```python
from build123d import *

# Parameters (mm, degrees)
SKETCH_1_R      = 1.75
SKETCH_1_R_2    = 1
EXTRUDE_1_DEPTH = 2.5
SKETCH_3_W      = 0.75
SKETCH_3_H      = 10
EXTRUDE_2_DEPTH = 0.75
SKETCH_4_W      = 10
SKETCH_4_H      = 0.75
EXTRUDE_3_DEPTH = 0.75


with BuildPart() as part:
    # 草图1 → 凸台-拉伸1 (new, symmetric)
    with BuildSketch(Plane.XY):
        Circle(SKETCH_1_R)
        Circle(SKETCH_1_R_2, mode=Mode.SUBTRACT)
    extrude(amount=EXTRUDE_1_DEPTH, both=True)

    # 草图3 → 凸台-拉伸2 (add)
    with BuildSketch(Plane.XY.offset(2.5)):
        with Locations((-1.375, -5)):
            Rectangle(SKETCH_3_W, SKETCH_3_H)
    extrude(amount=-EXTRUDE_2_DEPTH)

    # 草图4 → 凸台-拉伸3 (add)
    with BuildSketch(Plane(origin=(0, 0, -2.5), x_dir=(-1, 0, 0), z_dir=(0, 0, -1))):
        with Locations((-5, 1.375)):
            Rectangle(SKETCH_4_W, SKETCH_4_H)
    extrude(amount=-EXTRUDE_3_DEPTH)


solid = part.part
```
Work out the finished part from the listing and answer in its coordinate system (mm). Give positions to 0.01 mm unless a question says otherwise; leave off trailing zeros. Order: outer loops, then holes, each group sorted by start corner. A loop starts at its lowest first (then second) coordinate and runs counter-clockwise, first axis right, second up. Notation, with made-up numbers: M 1,30.25 L 34,30.25 A24 cw 34,49.25 Z; hole C 64.25,70.25 d6. An arc over 180 degrees is marked long. Return JSON: item names as keys, results as strings.
1) Section A-A, the plane z = 2.15 is taken. Write down the section's boundary in (x, y), plus the area to 3 significant figures.
Resolved:
{"outline": "M -1.75,-10 L -1,-10 L -1,-1.44 A1.75 ccw long -1.75,0 Z; hole C 0,0 d2", "area": "13.2 mm^2"}
2) For a pull along X with two mould halves and no side action, classify faces 1 (the flat face through (-1.2, -2.7, 2.5)), 2 (the cylindrical face through (0, -1, 0)) as +X half, -X half, draft (parallel to the pull), parting line (faces both ways), or undercut.
Resolved:
{"face 1": "draft", "face 2": "undercut"}
3) Each of these flat-tipped pins is pushed along its axis until it touches: pin 1 (1.5 mm diameter, centred on y = -0.5, z = 0.5, fed in from +X); pin 2 (0.8 mm diameter, centred on x = -1, y = -3, fed in from -Z); pin 3 (0.6 mm diameter, centred on y = -6, z = 2.5, fed in from +X). Where does it stop, or does it pass through?
Resolved:
{"pin 1": "x = 1.75", "pin 2": "z = 1.75", "pin 3": "x = -1"}
4) Straight lines are drawn through the part: line 1 along X through (y, z) = (0, 0.5); line 2 along X through (y, z) = (0.75, 1.05). For each, find the intervals that lie inside material, in ascending order. Write a range as [from, to].
Resolved:
{"line 1": "[-1.75, -1], [1, 1.75]", "line 2": "[-1.58, -0.66], [0.66, 1.58]"}
5) Section D-D, the plane y = -7.5 is taken. Write down the section's boundary in (x, z).
Resolved:
{"outline": "M -1.75,1.75 L -1,1.75 L -1,2.5 L -1.75,2.5 Z"}
6) Section C-C, the plane x = 2.25 is taken. Write down the section's boundary in (y, z).
Resolved:
{"outline": "M 1,-2.5 L 1.75,-2.5 L 1.75,-1.75 L 1,-1.75 Z"}
7) Section B-B, the plane y = 0.5 is taken. Write down the section's boundary in (x, z).
Resolved:
{"outline": "M -1.68,-2.5 L -0.87,-2.5 L -0.87,2.5 L -1.68,2.5 Z; M 0.87,-2.5 L 1.68,-2.5 L 1.68,2.5 L 0.87,2.5 Z"}
